Geometry: final body of the model. Coordinates: model frame, mm. Coordinates: 2 decimals unless noted, no trailing zeros. Write each loop counter-clockwise with the first axis right and the second up, starting at its lowest first coordinate (ties: lowest second). Pieces come first, ordered by that corner, then holes. Notation, with made-up numbers: (-23.75, 68) -> (-1.75, 68) arc R29 ccw to (-1.75, 107) -> close; hole circle Ø9 at (-0.75, 22). An arc over 180 degrees is marked (long way). One line per item, written item: value.
```python
from build123d import *

# Parameters (mm, degrees)
SKETCH1_W           = 110.344434204
SKETCH1_H           = 110.344434204
SKETCH1_R           = 1.6
SKETCH1_W_2         = 20.7
SKETCH1_H_2         = 41.4
BOSS_EXTRUDE1_DEPTH = 3
SKETCH3_W           = 3.2
SKETCH3_H           = 10.2
SKETCH3_W_2         = 10.2
SKETCH3_H_2         = 3.2
CUT_EXTRUDE1_DEPTH  = 4


with BuildPart() as part:
    # Sketch1 → Boss-Extrude1 (new body)
    with BuildSketch(Plane(origin=(0, 0, 0), x_dir=(1, 0, 0), z_dir=(0, 1, 0))):
        with Locations((0, -11.670773756)):
            Rectangle(SKETCH1_W, SKETCH1_H)
        with Locations((-5, 34.6)):
            Circle(SKETCH1_R, mode=Mode.SUBTRACT)
        with Locations((5, 34.6)):
            Circle(SKETCH1_R, mode=Mode.SUBTRACT)
        with Locations((5, -13.9)):
            Circle(SKETCH1_R, mode=Mode.SUBTRACT)
        with Locations((-5, -13.9)):
            Circle(SKETCH1_R, mode=Mode.SUBTRACT)
        with Locations((0, 10.35)):
            Rectangle(SKETCH1_W_2, SKETCH1_H_2, mode=Mode.SUBTRACT)
    extrude(amount=BOSS_EXTRUDE1_DEPTH)

    # Sketch3 → Cut-Extrude1 (cut, through all)
    with BuildSketch(Plane(origin=(0, 0, 0), x_dir=(1, 0, 0), z_dir=(0, 1, 0))):
        Polygon((-55.272217102, 43.601443346), (-55.272217102, 33.229226244), (-52.072217102, 33.229226244), (-52.072217102, 40.401443346), (-24.9, 40.401443346), (-24.9, 43.601443346), align=None)
        with Locations((-53.672217102, -1.670773756)):
            Rectangle(SKETCH3_W, SKETCH3_H)
        with Locations((-53.672217102, 18.329226244)):
            Rectangle(SKETCH3_W, SKETCH3_H)
        with Locations((-10, 42.001443346)):
            Rectangle(SKETCH3_W_2, SKETCH3_H_2)
        with Locations((-10, -65.342990858)):
            Rectangle(SKETCH3_W_2, SKETCH3_H_2)
        with Locations((-30, -65.342990858)):
            Rectangle(SKETCH3_W_2, SKETCH3_H_2)
        Polygon((-55.272217102, -56.570773756), (-52.072217102, -56.570773756), (-52.072217102, -63.742990858), (-44.9, -63.742990858), (-44.9, -66.942990858), (-55.272217102, -66.942990858), align=None)
        with Locations((-53.672217102, -21.670773756)):
            Rectangle(SKETCH3_W, SKETCH3_H)
        with Locations((-53.672217102, -41.670773756)):
            Rectangle(SKETCH3_W, SKETCH3_H)
        with Locations((30, -65.342990858)):
            Rectangle(SKETCH3_W_2, SKETCH3_H_2)
        with Locations((10, -65.342990858)):
            Rectangle(SKETCH3_W_2, SKETCH3_H_2)
        with Locations((53.672217102, -41.670773756)):
            Rectangle(SKETCH3_W, SKETCH3_H)
        with Locations((53.672217102, -21.670773756)):
            Rectangle(SKETCH3_W, SKETCH3_H)
        Polygon((52.072217102, -56.570773756), (52.072217102, -63.742990858), (44.9, -63.742990858), (44.9, -66.942990858), (55.272217102, -66.942990858), (55.272217102, -56.570773756), align=None)
        with Locations((53.672217102, -1.670773756)):
            Rectangle(SKETCH3_W, SKETCH3_H)
        with Locations((53.672217102, 18.329226244)):
            Rectangle(SKETCH3_W, SKETCH3_H)
        Polygon((24.9, 43.601443346), (24.9, 40.401443346), (52.072217102, 40.401443346), (52.072217102, 33.229226244), (55.272217102, 33.229226244), (55.272217102, 43.601443346), align=None)
        with Locations((10, 42.001443346)):
            Rectangle(SKETCH3_W_2, SKETCH3_H_2)
    extrude(amount=CUT_EXTRUDE1_DEPTH, mode=Mode.SUBTRACT)


solid = part.part
```
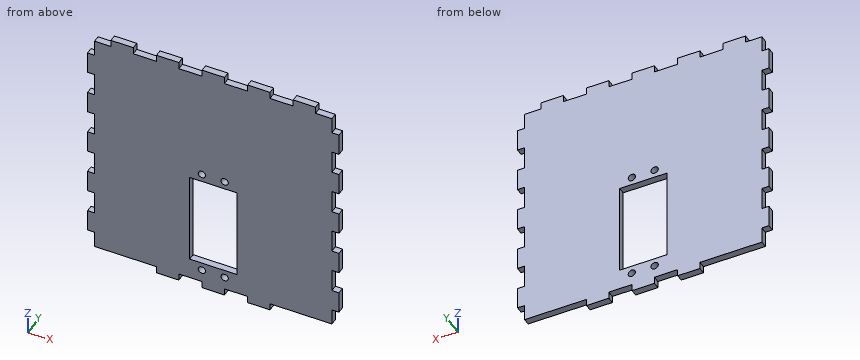
(1) Line query: line 1 (Z direction, x = 5, y = 1.8); line 2 (X direction, y = 1.3, z = 13.9); line 3 (X direction, y = 1, z = -34.6). Output: solid intervals per line, ascending. Write a range as [from, to].
Responses:
line 1: z = [-40.4, -36.2], [-33, -31.05], [10.35, 12.3], [15.5, 63.74]
line 2: x = [-55.17, -6.6], [-3.4, 3.4], [6.6, 55.17]
line 3: x = [-52.07, -6.6], [-3.4, 3.4], [6.6, 52.07]
(2) First-contact query: pin 1 (1.5 mm diameter, centred on x = -32, y = 1.5, fed in from +Z); pin 2 (0.9 mm diameter, centred on y = 1.5, z = 65.5, fed in from -X); pin 3 (0.9 mm diameter, centred on y = 1, z = -42.5, fed in from +X). Flat tips, straight axial feed; report the tip coordinate or a pass-through.
Responses:
pin 1: stops at z = 63.74
pin 2: stops at x = -44.9
pin 3: stops at x = 24.9
(3) Section A-A (z = -34.6). Return the cut outline in (x, y).
Responses:
outline: (-52.07, 0) -> (-6.6, 0) -> (-6.6, 3) -> (-52.07, 3) -> close; (-3.4, 0) -> (3.4, 0) -> (3.4, 3) -> (-3.4, 3) -> close; (6.6, 0) -> (52.07, 0) -> (52.07, 3) -> (6.6, 3) -> close
(4) Section C-C (x = 0). Return the cut outline in (y, z), then the cut area to 3 significant figures.
Responses:
outline: (0, -43.5) -> (3, -43.5) -> (3, -31.05) -> (0, -31.05) -> close; (0, 10.35) -> (3, 10.35) -> (3, 66.84) -> (0, 66.84) -> close
area: 207 mm2
(5) Section D-D (z = 13.9). Return the cut outline in (x, y).
Responses:
outline: (-55.17, 0) -> (-6.6, 0) -> (-6.6, 3) -> (-55.17, 3) -> close; (-3.4, 0) -> (3.4, 0) -> (3.4, 3) -> (-3.4, 3) -> close; (6.6, 0) -> (55.17, 0) -> (55.17, 3) -> (6.6, 3) -> close
(6) Section B-B (z = -6). Return the cut outline in (x, y).
Responses:
outline: (-55.17, 0) -> (-10.35, 0) -> (-10.35, 3) -> (-55.17, 3) -> close; (10.35, 0) -> (55.17, 0) -> (55.17, 3) -> (10.35, 3) -> close
